Here's how the part is built. I have some questions about the finished solid (model axes, mm). A direction names the side the tool comes from. Round coordinates to 2 decimals unless told otherwise and drop trailing zeros. Use a Markdown table: item, result. Add a question column.
```python
from build123d import *

# Parameters (mm, degrees)
F1_DEPTH = 2
F2_SIZE  = 1.99999
F4_D     = 6


# Not quite as in the source:
# - a fillet or chamfer is up to 0.001 mm smaller than in the source, because OpenCascade refuses the exact size


with BuildPart() as f1:
    # F0 (on Top) → F1 (new body)
    with BuildSketch(Plane.XY):
        with BuildLine():
            Line((-6.070732047, 22.9513901076), (-7.1661561031, 9.2087939751))
            add(Edge.make_bspline(
                [(-10.8183338371, 4.072241369), (-9.5749830205, 3.3108681768), (-7.3147246833, 1.9267856777), (-3.6193330593, 2.323879706), (-3.8736126343, 6.3110586072), (-5.9992796786, 8.181837424), (-7.1661561031, 9.2087939751)],
                knots=[0, 0, 0, 0, 0.2710094176, 0.4926616748, 0.721498655, 1, 1, 1, 1], degree=3))
            Line((-10.8183338371, 4.072241369), (-23.7063266087, -0.9532651191))
            Line((-23.7063266087, -0.9532651191), (-10.4941075873, -5.6545452478))
            add(Edge.make_bspline(
                [(-10.4941075873, -5.6545452478), (-9.4938612527, -5.0046237284), (-7.5990391104, -3.7734413255), (-4.2858275376, -3.7917280391), (-3.3433653275, -6.5786033893), (-4.5476101592, -8.3403208195), (-5.9073550155, -9.6570884675), (-6.7070025438, -10.4037433444), (-7.0897310874, -10.7611084628)],
                knots=[0, 0, 0, 0, 0.2047671487, 0.3879017737, 0.5554252257, 0.7107538026, 0.8615605352, 1, 1, 1, 1], degree=3))
            Line((-7.0897310874, -10.7611084628), (-6.0359964333, -24.702837204))
            Line((-6.0359964333, -24.702837204), (2.1507161547, -13.8412582744))
            add(Edge.make_bspline(
                [(2.1507161547, -13.8412582744), (1.857437852, -12.3709258177), (1.3508773092, -9.8313161697), (2.3957995803, -7.6684734808), (3.0110019697, -6.7670125475), (5.8159743775, -7.4801379246), (7.4501009355, -10.1557150048), (7.8283613318, -11.2679488073), (7.9867886511, -11.7337872122)],
                knots=[0, 0, 0, 0, 0.2247705341, 0.3882315284, 0.4906474402, 0.664362762, 0.8594245965, 1, 1, 1, 1], degree=3))
            Line((7.9867886511, -11.7337872122), (21.4421775791, -15.3813331802))
            Line((21.4421775791, -15.3813331802), (13.4529346897, -3.7091881875))
            add(Edge.make_bspline(
                [(13.4529346897, 1.9505254996), (11.9323407983, 1.79071702), (9.5330178877, 1.5385575522), (8.581661333, 0.6216498394), (6.8511425341, -1.0519539126), (9.4923390362, -3.4928584716), (12.2268542531, -3.6020610918), (13.107191535, -3.6789793538), (13.4529346897, -3.7091881875)],
                knots=[0, 0, 0, 0, 0.2219857691, 0.3502681055, 0.5009951592, 0.691693444, 0.8789158616, 1, 1, 1, 1], degree=3))
            Line((13.4529346897, 1.9505254996), (21.5007144708, 13.33170683))
            Line((21.5007144708, 13.33170683), (8.0718742184, 9.9506860604))
            add(Edge.make_bspline(
                [(2.294327212, 12.4950657049), (2.1198852992, 10.9346638034), (1.8320041162, 8.3595352793), (1.8961121506, 6.5524820747), (3.1599495173, 4.614552865), (6.0828787964, 6.0160070097), (7.1855048229, 8.2606927811), (7.7920128495, 9.4170893061), (8.0718742184, 9.9506860604)],
                knots=[0, 0, 0, 0, 0.2205766948, 0.364017333, 0.5063227579, 0.6820195585, 0.8532740908, 1, 1, 1, 1], degree=3))
            Line((2.294327212, 12.4950657049), (-6.070732047, 22.9513901076))
        make_face()
    extrude(amount=F1_DEPTH)

    # F2 (size 2 in the source; OpenCascade refuses exactly that, so slightly less here)
    f2_edges = [f1.edges().sort_by_distance(p)[0] for p in [
        (-1.888202, 17.723228, 2),
        (-6.618444, 16.080092, 2),
        (17.476825, 7.641116, 2),
        (14.786294, 11.641196, 2),
        (17.447556, -9.545261, 2),
        (14.714483, -13.55756, 2),
        (-1.94264, -19.272048, 2),
        (-6.562864, -17.731973, 2),
        (-17.100217, -3.303905, 2),
        (-17.26233, 1.559488, 2),
    ]]
    chamfer(f2_edges, length=F2_SIZE)

    # F4 (through all)
    with Locations(Plane(origin=(0, 0, 0), x_dir=(1, 0, 0), z_dir=(0, 0, -1))):
        with Locations((1.6917608845, 0.5521112873)):
            Hole(F4_D / 2)


solid = f1.part
```
Item 1: For pin 1 Ø1 at (y, z) = (-10, 1) entering from -X; pin 2 Ø8 at (x, y) = (4, 1.5) entering from -Z, each with a flat end and sliding along its axis, tell me the tip position at first contact or that it passes through.
Item 2: On a 3-axis mill with a long thin cutter (end or side, diameter ignored), from which of +Z, -Z, +X, -X, +Y, -Y can I reach the whole of each face in a straight line? I mean faces 5 (the face through (-14.41, -3.19, 1.01)), 6 (the face through (16.06, 7.39, 1.01)). Say none if no direction works.
Item 3: I need wall thicknesses on probe 1 along Y at (x, z) = (-4.5, 1.05); probe 2 along Y at (x, z) = (11.5, 1.2); probe 3 along Y at (x, z) = (-1, 1.4). Which ranges of each line are inside material? Lowest first, please. Write a range as from..to.
Item 4: If we mould it in two halves opening along X, with no side actions, what happens to faces 1 (the face through (-1, -3, 2)), 2 (the face through (15.22, -8.08, 1.01)), 3 (the face through (12.596, 10.044, 1.014)), 4 (the face through (-16.026, 0.953, 1.014))? For each: +X half, -X half, draft (parallel to the pull), parting line (faces both ways), or undercut.
The answers:
| question | item | result |
|---|---|---|
| 1 | pin 1 | x = -6.55 |
| 1 | pin 2 | z = 0 |
| 2 | face 5 | +Z, -X, -Y |
| 2 | face 6 | +Z, +X |
| 3 | probe 1 | -20.92..-8.18, -4.38..2.62, 6.34..19.31 |
| 3 | probe 2 | -11.44..-3.56, 1.73..9.58 |
| 3 | probe 3 | -15.7..-1.88, 0.77..14.37 |
| 4 | face 1 | draft |
| 4 | face 2 | +X half |
| 4 | face 3 | undercut |
| 4 | face 4 | -X half |
